from build123d import *

# Parameters (mm, degrees)
SKETCH1_W           = 103
SKETCH1_H           = 74
BOSS_EXTRUDE2_DEPTH = 3
SKETCH1_12_R        = 1.35
CUT_EXTRUDE1_DEPTH  = 3
FILLET1_R           = 4


with BuildPart() as part:
    # Sketch1 → Boss-Extrude2 (new body)
    with BuildSketch(Plane.YZ):
        with Locations((10, 0)):
            Rectangle(SKETCH1_W, SKETCH1_H)
    extrude(amount=-BOSS_EXTRUDE2_DEPTH)

    # Sketch1_12 → Cut-Extrude1 (cut)
    with BuildSketch(Plane.YZ):
        with Locations(Location((-29, 24.5, 0), (0, 0, 270))):
            Circle(SKETCH1_12_R)
        with Locations(Location((-29, -24.5, 0), (0, 0, 270))):
            Circle(SKETCH1_12_R)
        with Locations(Location((29, -24.5, 0), (0, 0, 270))):
            Circle(SKETCH1_12_R)
        with Locations(Location((29, 24.5, 0), (0, 0, 90))):
            Circle(SKETCH1_12_R)
    extrude(amount=-CUT_EXTRUDE1_DEPTH, mode=Mode.SUBTRACT)

    # Fillet1
    fillet1_edges = [part.edges().sort_by_distance(p)[0] for p in [
        (-1.5, 61.5, 37),
        (-1.5, 61.5, -37),
        (-1.5, -41.5, -37),
        (-1.5, -41.5, 37),
    ]]
    fillet(fillet1_edges, radius=FILLET1_R)


solid = part.part
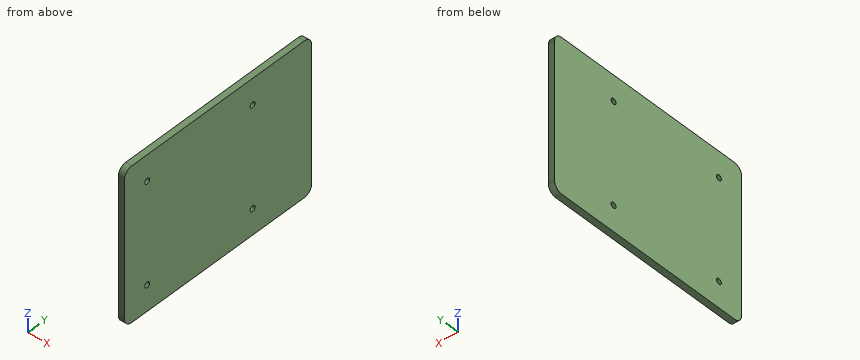
Design review of the part built by this model. Coordinates are the model's own, in mm. Give positions to 0.01 mm unless a question says otherwise; leave off trailing zeros. Loops run counter-clockwise (first coordinate to the right, second up) from the corner with the lowest first, then second, coordinate; pieces in that order, holes last. Notation, with made-up numbers: M 88,-3.75 L 110,-3.75 A20 ccw 110,4.25 Z; hole C 25,-27.5 d3. An arc over 180 degrees is marked long. Answer as a JSON object with one key per item and string values.
Item 1: For P1, Ø1.5, axis at y = -1.5, z = -18.5, coming from the +X side; P2, Ø2.5, axis at y = -29, z = -24.5, coming from the -X side, all flat-tipped, find the tip position at first contact; note any pin that passes through.
Output values:
{"P1": "stops at x = 0", "P2": "passes through"}
Item 2: We need section A-A (y = 29). State the section outline as (x, z) points, and give its area (3 significant figures).
Output values:
{"outline": "M -3,-37 L 0,-37 L 0,-25.85 L -3,-25.85 Z; M -3,-23.15 L 0,-23.15 L 0,23.15 L -3,23.15 Z; M -3,25.85 L 0,25.85 L 0,37 L -3,37 Z", "area": "206 mm2"}
Item 3: Wall thickness on line 1 along Y through (x, z) = (-2.4, 24.5): over which ranges is the line inside the solid? List them lowest first.
Output values:
{"line 1": "y = -41.5 to -30.35, -27.65 to 27.65, 30.35 to 61.5"}
Item 4: We need section B-B (z = 24.5). State the section outline as (x, y) points.
Output values:
{"outline": "M -3,-41.5 L 0,-41.5 L 0,-30.35 L -3,-30.35 Z; M -3,-27.65 L 0,-27.65 L 0,27.65 L -3,27.65 Z; M -3,30.35 L 0,30.35 L 0,61.5 L -3,61.5 Z"}
